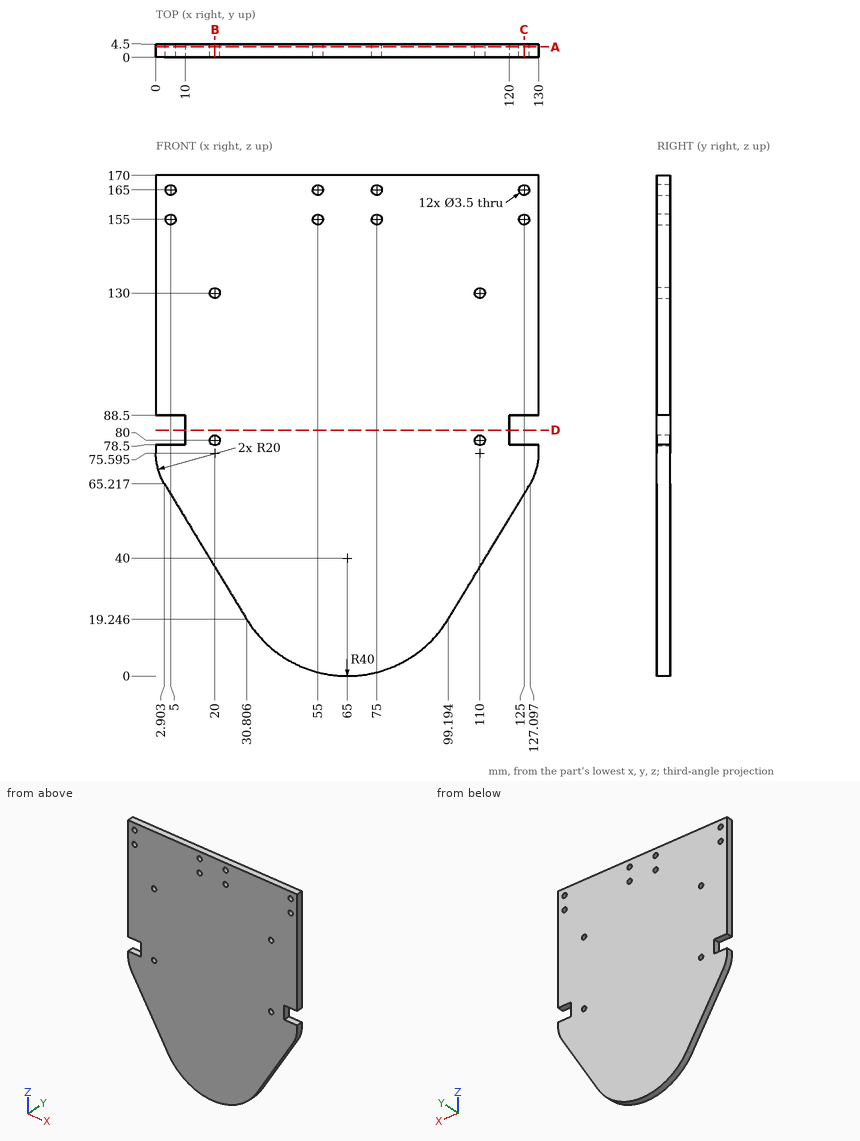
Drawing for the job (mm, zero at the part's lowest x, y, z). Round coordinates to 2 decimals unless told otherwise and drop trailing zeros. Loops run counter-clockwise (first coordinate to the right, second up) from the corner with the lowest first, then second, coordinate; pieces in that order, holes last. Notation, with made-up numbers: (12, 10) - (49, 10) arc R26 cw to (49, 41) - close; hole circle Ø11 at (36.25, 50.25). An arc over 180 degrees is marked (long way). Return JSON: item names as keys, results as strings. Group by question number.
Q1. Drill centre lines: line 1 along X through (y, z) = (2.85, 130); line 2 along Z through (x, y) = (54.5, 3.95); line 3 along Z through (x, y) = (75, 3). Where is each one in solid material? Low to high. Write a range as [from, to].
Q2. Band-saw the part on C-C on x = 125. Give the cut face in (y, z).
Q3. Band-saw the part on B-B on x = 20. Give the cut face in (y, z), plus the area to 3 significant figures.
Q4. Flat gauge pins, fed straight in: pin 1 Ø1.5 at (x, y) = (27, 2.5) entering from -Z; pin 2 Ø2 at (x, y) = (4.5, 2.5) entering from -Z. Where does each tip first touch, or does it go through?
Q5. Band-saw the part on D-D on z = 83.5. Give the cut face in (x, y), plus the area to 3 significant figures.
Q6. Band-saw the part on A-A on y = 3.5. Give the number of separate pieces and of enclosed holes in the cut face, plus the area to 3 significant figures.
Solutions:
{
 "1": {"line 1": "x = [0, 18.25], [21.75, 108.25], [111.75, 130]", "line 2": "z = [1.4, 153.32], [156.68, 163.32], [166.68, 170]", "line 3": "z = [1.27, 153.25], [156.75, 163.25], [166.75, 170]"},
 "2": {"outline": "(0, 61.76) - (4.5, 61.76) - (4.5, 78.5) - (0, 78.5) - close; (0, 88.5) - (4.5, 88.5) - (4.5, 153.25) - (0, 153.25) - close; (0, 156.75) - (4.5, 156.75) - (4.5, 163.25) - (0, 163.25) - close; (0, 166.75) - (4.5, 166.75) - (4.5, 170) - (0, 170) - close"},
 "3": {"outline": "(0, 37.05) - (4.5, 37.05) - (4.5, 78.25) - (0, 78.25) - close; (0, 81.75) - (4.5, 81.75) - (4.5, 128.25) - (0, 128.25) - close; (0, 131.75) - (4.5, 131.75) - (4.5, 170) - (0, 170) - close", "area": "567 mm^2"},
 "4": {"pin 1": "stops at z = 24.28", "pin 2": "stops at z = 60.94"},
 "5": {"outline": "(10, 0) - (120, 0) - (120, 4.5) - (10, 4.5) - close", "area": "495 mm^2"},
 "6": {"separate pieces": "1", "enclosed holes": "12", "area": "18,600 mm^2"}
}
